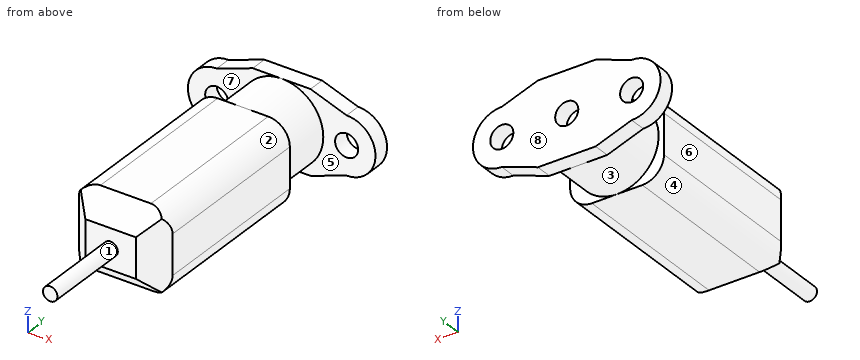
```python
from build123d import *

# Parameters (mm, degrees)
SKETCH1_R           = 1.6
BOSS_EXTRUDE1_DEPTH = 2.3
SKETCH2_R           = 5.765
BOSS_EXTRUDE2_DEPTH = 7.7
SKETCH3_W           = 13
SKETCH3_H           = 11.53
BOSS_EXTRUDE3_DEPTH = 26.3
SKETCH4_R           = 1
BOSS_EXTRUDE4_DEPTH = 12
CHAMFER1_SIZE       = 3
FILLET1_R           = 3


with BuildPart() as part:
    # Sketch1 → Boss-Extrude1 (new body)
    with BuildSketch(Plane.XZ.offset(2.3)):
        with BuildLine():
            Line((-75.699998599, -20.764999665), (-67.699998599, -20.764999665))
            Line((-67.699998599, -20.764999665), (-62.699998599, -18.999999665))
            ThreePointArc((-62.699998599, -18.999999665), (-58.699998599, -14.999999665), (-62.699998599, -10.999999665))
            Line((-62.699998599, -10.999999665), (-67.699998599, -9.234999665))
            Line((-67.699998599, -9.234999665), (-75.699998599, -9.234999665))
            Line((-75.699998599, -9.234999665), (-80.699998599, -10.999999665))
            ThreePointArc((-80.699998599, -10.999999665), (-84.699998599, -14.999999665), (-80.699998599, -18.999999665))
            Line((-80.699998599, -18.999999665), (-75.699998599, -20.764999665))
        make_face()
        with Locations((-62.699998599, -14.999999665)):
            Circle(SKETCH1_R, mode=Mode.SUBTRACT)
        with Locations((-71.699998599, -14.999999665)):
            Circle(SKETCH1_R, mode=Mode.SUBTRACT)
        with Locations((-80.699998599, -14.999999665)):
            Circle(SKETCH1_R, mode=Mode.SUBTRACT)
    extrude(amount=-BOSS_EXTRUDE1_DEPTH)

    # Sketch2 → Boss-Extrude2 (add)
    with BuildSketch(Plane.XZ.offset(2.3)):
        with Locations((-71.699998599, -14.999999665)):
            Circle(SKETCH2_R)
    extrude(amount=BOSS_EXTRUDE2_DEPTH)

    # Sketch3 → Boss-Extrude3 (add)
    with BuildSketch(Plane.XZ.offset(10)):
        with Locations((-71.699998599, -14.999999665)):
            Rectangle(SKETCH3_W, SKETCH3_H)
    extrude(amount=BOSS_EXTRUDE3_DEPTH)

    # Sketch4 → Boss-Extrude4 (add)
    with BuildSketch(Plane.XZ.offset(36.3)):
        with Locations((-71.699998599, -14.999999665)):
            Circle(SKETCH4_R)
    extrude(amount=BOSS_EXTRUDE4_DEPTH)

    # Chamfer1
    chamfer1_edges = [part.edges().sort_by_distance(p)[0] for p in [
        (-71.699998599, -36.3, -9.234999665),
        (-78.199998599, -36.3, -14.999999665),
        (-71.699998599, -36.3, -20.764999665),
        (-65.199998599, -36.3, -14.999999665),
    ]]
    chamfer(chamfer1_edges, length=CHAMFER1_SIZE)

    # Fillet1
    fillet1_edges = [part.edges().sort_by_distance(p)[0] for p in [
        (-78.199998599, -21.65, -20.764999665),
        (-78.199998599, -21.65, -9.234999665),
        (-65.199998599, -21.65, -9.234999665),
        (-65.199998599, -21.65, -20.764999665),
    ]]
    fillet(fillet1_edges, radius=FILLET1_R)


solid = part.part
```
Source: CAD feature listing. Evaluate the final solid. Frame: model axes, mm. Face numbers are marked on the shaded views. A direction names the side the tool comes from. Round coordinates to 2 decimals unless told otherwise and drop trailing zeros. Loops run counter-clockwise (first coordinate to the right, second up) from the corner with the lowest first, then second, coordinate; pieces in that order, holes last. Notation, with made-up numbers: M 77.25,59.25 L 133.25,59.25 A20 ccw 133.25,69.25 Z; hole C 47.25,-7 d3. An arc over 180 degrees is marked long. Use a Markdown table: item, result. Add a question column.
1. Mould query, pull axis Y, two halves, no side actions, for the marked faces 5, 6, 7 and 8. Classes: pulls with the +Y half, pulls with the -Y half, needs draft (parallel to the pull), parting line crosses it, or undercut.
2. Section query A-A on z = -15. Give the number of separate pieces and of enclosed holes in the cut face, then the cut area to 3 significant figures.
3. Section query B-B on y = -22.5. Return the cut outline in (x, z) (3 decimals).
4. Contact query for flat-ended pins moving along their axis: P1, Ø2.5, axis at x = -80.7, z = -15, coming from the -Y side; P2, Ø6, axis at x = -64.5, y = -6.5, coming from the -Z side; P3, Ø3, axis at x = -75, z = -13.5, coming from the -Y side; P4, Ø2, axis at y = -26, z = -15, coming from the -X side. Output: stop coordinate, or through.
5. Section query C-C on x = -76.5. Return the cut outline in (y, z) (3 decimals).
6. Reachability of the marked faces 1, 2, 3 and 4 from +Z, -Z, +X, -X, +Y, -Y: full face, straight path, thin tool, end or side. Return the list, or none.
7. Section query D-D on z = -17.25. Return the cut outline in (x, y).
8. Line query: line 1 (X direction, y = -28.5, z = -15); line 2 (Y direction, x = -65.25, z = -10.5); line 3 (Y direction, x = -68.5, z = -15.75). Output: solid intervals per line, ascending.
Reported:
| question | item | result |
|---|---|---|
| 1 | face 5 | undercut |
| 1 | face 6 | needs draft |
| 1 | face 7 | undercut |
| 1 | face 8 | pulls with the +Y half |
| 2 | separate pieces | 3 |
| 2 | enclosed holes | 0 |
| 2 | area | 483 mm² |
| 3 | outline | M -78.2,-17.765 A3 ccw -75.2,-20.765 L -68.2,-20.765 A3 ccw -65.2,-17.765 L -65.2,-12.235 A3 ccw -68.2,-9.235 L -75.2,-9.235 A3 ccw -78.2,-12.235 Z |
| 4 | P1 | passes through |
| 4 | P2 | stops at z = -18.95 |
| 4 | P3 | stops at y = -36.3 |
| 4 | P4 | stops at x = -78.2 |
| 5 | outline | M -35,-19.065 L -33.596,-20.469 L -10,-20.469 L -10,-18.193 L -2.3,-18.193 L -2.3,-20.483 L 0,-20.483 L 0,-9.517 L -2.3,-9.517 L -2.3,-11.807 L -10,-11.807 L -10,-9.531 L -33.596,-9.531 L -35,-10.935 Z |
| 6 | face 1 | -Y |
| 6 | face 2 | +Z, +X, -Y |
| 6 | face 3 | none |
| 6 | face 4 | -Z, -X, -Y |
| 7 | outline | M -84.01,-2.3 L -77.01,-2.3 L -77.01,-10 L -78.2,-10 L -78.2,-33.3 L -75.2,-36.3 L -68.2,-36.3 L -65.2,-33.3 L -65.2,-10 L -66.39,-10 L -66.39,-2.3 L -59.39,-2.3 L -59.39,0 L -84.01,0 Z |
| 8 | line 1 | x = -78.2 to -65.2 |
| 8 | line 2 | y = -2.3 to 0 |
| 8 | line 3 | y = -36.3 to 0 |
